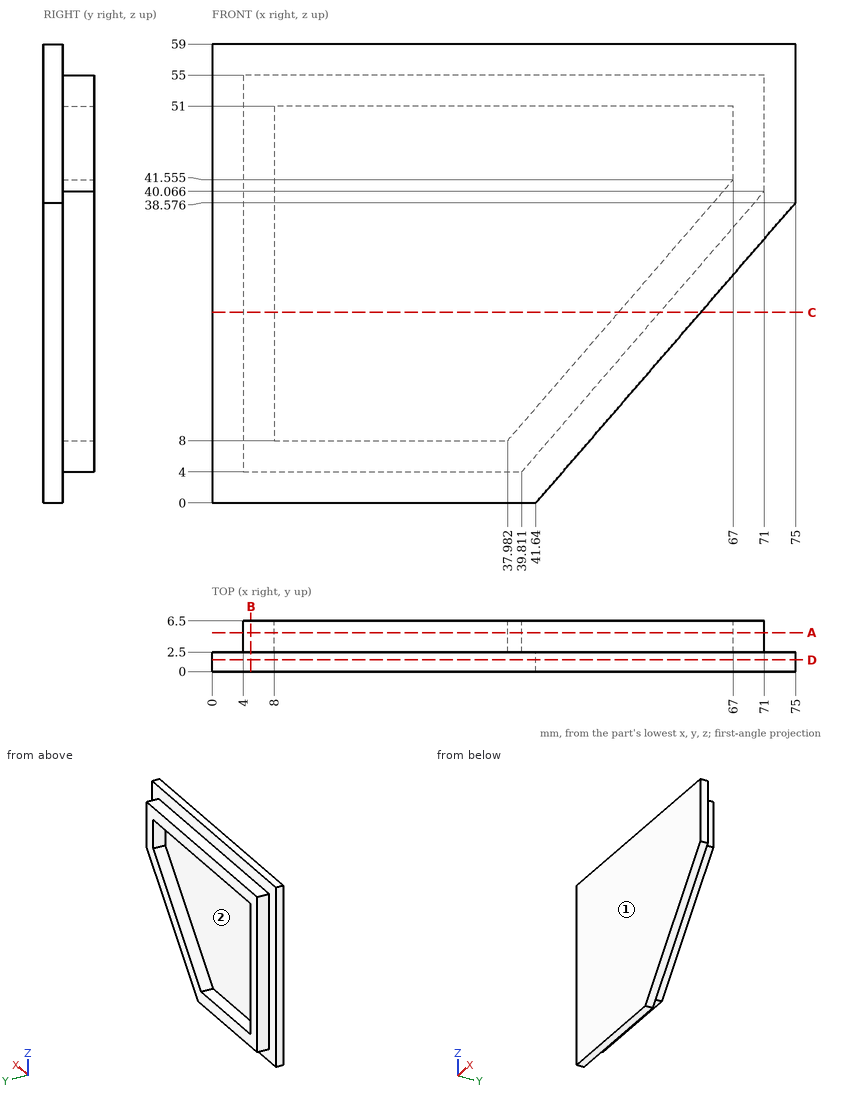
Job drawing, mm, ordinate dimensions from the low corner. One solid piece. Round coordinates to 2 decimals unless told otherwise and drop trailing zeros. Loops run counter-clockwise (first coordinate to the right, second up) from the corner with the lowest first, then second, coordinate; pieces in that order, holes last. Notation, with made-up numbers: (32.5, 72.5) -> (60.5, 72.5) arc R5 ccw to (60.5, 80.5) -> close; hole circle Ø7 at (13, -30). An arc over 180 degrees is marked (long way). One line per item, written item: value. Start each with the question number.
Q1. Cut at D-D on y = 1.5. List the corners of the cut face in (x, z), plus the area to 3 significant figures.
Q2. Probe line 1 along X through (y, z) = (4.5, 44); line 2 along Z through (x, y) = (20, 3.5); line 3 along Y through (x, z) = (36.5, 35). List the from-to ranges inside material, lowest first.
Q3. Drop flat-ended pins along their axis: pin 1 Ø1.2 at (x, y) = (24, 3.5) entering from -Z; pin 2 Ø2 at (y, z) = (4, 48) entering from -X; pin 3 Ø3 at (y, z) = (4.5, 47) entering from +X. Give the stop position or say it passes through.
Q4. Two-plate mould, pull along X, no slides. Class the marked faces 1 and 2: released by +X, released by -X, zero draft, split by the parting line, or undercut.
Q5. Cut at B-B on x = 5. List the corners of the cut face in (y, z).
Q6. Cut at C-C on z = 24.5. List the corners of the cut face in (x, y).
Q7. Cut at A-A on y = 5. List the corners of the cut face in (x, z) (1 decimal).
Computed:
1. outline: (0, 0) -> (41.64, 0) -> (75, 38.58) -> (75, 59) -> (0, 59) -> close
1. area: 3,780 mm²
2. line 1: 4 to 8, 67 to 71
2. line 2: 4 to 8, 51 to 55
2. line 3: 0 to 2.5
3. pin 1: z = 4
3. pin 2: x = 4
3. pin 3: x = 71
4. face 1: zero draft
4. face 2: undercut
5. outline: (0, 0) -> (2.5, 0) -> (2.5, 4) -> (6.5, 4) -> (6.5, 55) -> (2.5, 55) -> (2.5, 59) -> (0, 59) -> close
6. outline: (0, 0) -> (62.83, 0) -> (62.83, 2.5) -> (57.54, 2.5) -> (57.54, 6.5) -> (52.25, 6.5) -> (52.25, 2.5) -> (8, 2.5) -> (8, 6.5) -> (4, 6.5) -> (4, 2.5) -> (0, 2.5) -> close
7. outline: (4, 4) -> (39.8, 4) -> (71, 40.1) -> (71, 55) -> (4, 55) -> close; hole (8, 8) -> (38, 8) -> (67, 41.6) -> (67, 51) -> (8, 51) -> close
